Input: part model. Units: mm. Frame: model coordinates. Face numbers are marked on the shaded views. A direction names the side the tool comes from. Coordinates: 2 decimals unless noted, no trailing zeros. Loops run counter-clockwise (first coordinate to the right, second up) from the corner with the lowest first, then second, coordinate; pieces in that order, holes last. Notation, with made-up numbers: (26, -24) -> (77, -24) arc R36 ccw to (77, 13) -> close; hole circle Ø5 at (17, -23). An arc over 180 degrees is marked (long way). Put each result on its own line as item: value. Start each with the question number.
1) Contact query for flat-ended pins moving along their axis: P1, Ø7.5, axis at y = 9.5, z = 14.5, coming from the -X side; P2, Ø0.6, axis at x = 0, y = 8, coming from the -Z side; P3, Ø2, axis at x = 0, y = 4.5, coming from the -Z side; P4, Ø0.7, axis at x = -2, y = 6.5, coming from the +Z side. Output: stop coordinate, or through.
2) Material intervals for L1, parallel to Z at x = -2.05, y = 9.25; L2, parallel to Z at x = -0.75, y = 8.25; L3, parallel to X at y = 1.75, z = 7.5, sorted ascending.
3) Cut plane A-A (z = -7.5). Return the cut outline in (x, y), plus the area to 3 significant figures.
4) Pull-direction query (Z, two-part tool) for the marked faces 3, 4, 5 and 6; classes: pulls with the +Z half, pulls with the -Z half, needs draft (parallel to the pull), parting line crosses it, or undercut.
5) Set-up query: the marked faces 1 and 2. Return all of +Z, -Z, +X, -X, +Y, -Y with unobstructed straight access to the full face (end or side cutting, diameter ignored); none if empty.
Autodesk Inventor part; units mm, degrees
ref_plane "YZ Plane" through (0, 0, 0) normal (1, 0, 0) x (0, 1, 0)
ref_plane "XZ Plane" through (0, 0, 0) normal (0, 1, 0) x (-1, 0, 0)
ref_plane "XY Plane" through (0, 0, 0) normal (0, 0, 1) x (1, 0, 0)
sketch "Skizze1" plane through (0, 0, 0) normal (0, 1, 0) x (-1, 0, 0)
  line L0 (1.2301, 16.646) -> (-1.7699, 16.646)
  line L1 (-1.7699, 16.646) -> (-1.7699, 9.646)
  line L2 (-1.7699, 9.646) -> (1.2301, 9.646)
  line L3 (1.2301, 9.646) -> (1.2301, 16.646)
  line L4 (-1.7699, 9.646) -> (-0.5699, 9.646)
  line L5 (-0.5699, 9.646) -> (-0.5699, -20.354)
  line L6 (-0.5699, -20.354) -> (-1.7699, -20.354)
  line L7 (-1.7699, -20.354) -> (-1.7699, 9.646)
  line L8 (-0.5699, -20.354) -> (3.4301, -20.354)
  line L9 (3.4301, -20.354) -> (3.4301, -15.9771)
  line L10 (3.4301, -15.9771) -> (-0.5699, -15.9771)
  line L11 (-0.5699, -15.9771) -> (-0.5699, -20.354)
  point P0 (0, 0)
  dimension "d0" = 3
  dimension "d1" = 7
  dimension "d2" = 1.2
  dimension "d3" = 30
  dimension "d4" = 4
extrude "Extrusion1" add sketch "Skizze1" along normal blind 13
fillet "Rundung1" radius 4 1 edges at (1.7699, 6.5, -20.354)
sketch "Skizze2" plane through (0, 13, 0) normal (0, 1, 0) x (1, 0, 0)
  line L0 (0.5699, -9.646) -> (-1.2301, -9.646)
  line L1 (0.5699, -9.646) -> (-0.1301, -9.646)
  line L2 (-0.1301, -9.646) -> (-0.1301, -14.642)
  line L3 (-0.1301, -14.642) -> (0.5699, -14.642)
  line L4 (0.5699, -14.642) -> (0.5699, -9.646)
  point P0 (0, 0)
  point P1 (-0.3301, -9.646)
  point P2 (-0.1301, -9.646)
  dimension "d8" = 5
  dimension "d9" = 0.7
sketch "Skizze3" plane through (0, 13, 0) normal (0, 1, 0) x (1, 0, 0)
  line L0 (-3.4301, 20.354) -> (-3.4301, 15.9771)
  line L1 (-3.4301, 15.9771) -> (0.5699, 15.9771)
  arc A0 (0.5699, 15.9771) -> (-2.5715, 19.8839) centre (-3.4301, 15.9771) ccw
  line L2 (0.5699, 15.9771) -> (0.5699, -9.646)
  line L3 (0.5699, 15.9771) -> (-0.0301, 15.9771)
  arc A1 (-0.0301, 15.9771) -> (-2.8554, 19.3282) centre (-3.4301, 15.9771) ccw
  line L4 (-2.8554, 19.3282) -> (-2.5715, 19.8839)
  point P0 (0, 0)
  dimension "d10" = 0.6
extrude "Extrusion2" cut sketch "Skizze3" against normal blind 12
extrude "Extrusion3" cut sketch "Skizze2" against normal blind 12
sketch "Skizze4" plane through (-1.2301, 0, 9.646) normal (-1, 0, 0) x (0, 0, 1)
  line L0 (0, 0) -> (7, 0)
  line L1 (7, 0) -> (3.5, 0)
  line L2 (4.996, 13) -> (0, 13)
  line L3 (3.5, 13) -> (3.5, 0)
  line L4 (3.5, 6.5) -> (7, 6.5)
  line L5 (7, 0) -> (7, 13)
  circle A0 centre (3.5, 6.5) radius 1
  circle A1 centre (3.5, 1.1664) radius 1
  circle A2 centre (3.5, 3.7221) radius 1
  circle A3 centre (3.5, 8.9382) radius 1
  circle A4 centre (3.5, 11.2973) radius 1
  point P0 (-9.646, 0)
  dimension "d15" = 2
  dimension "d16" = 2
  dimension "d17" = 2
  dimension "d18" = 2
  dimension "d19" = 2
extrude "Extrusion4" add sketch "Skizze4" along normal blind 2.5 contours A4 L3 | L3 A4 | A3 L3 | L3 A3 | A1 L3 | L3 A1 | A0 L3 L4 | L4 L3 A0 | A2 L3 | L3 A2 | L3 A0
ref_plane "Arbeitsebene1" through (-1.2301, 11.2973, 14.146) normal (0, 0, 1) x (1, 0, 0)
sketch "Skizze5" plane through (-1.2301, 11.2973, 14.146) normal (0, 0, 1) x (1, 0, 0)
  line L0 (-2.2, -11.2973) -> (-2.2, 1.7027)
  ellipse E0 centre (-0.7, -4.7973) end of major axis (-0.7, -3.6152) minor radius 0.3015
  ellipse E1 centre (-0.7, -2.3523) end of major axis (-0.7, -1.125) minor radius 0.2616
  line L1 (0, -1.3591) -> (-2.5, -1.3591)
  ellipse E2 centre (-0.7, 0.0155) end of major axis (-0.7, 1.1416) minor radius 0.2973
  circle A0 centre (-1.25, -10.1312) radius 0.3762
  ellipse E3 centre (-0.7, -7.4834) end of major axis (-0.7, -8.7492) minor radius 0.3
  line L2 (0, -8.5752) -> (-2.5, -8.5752)
  point P0 (1.2301, -11.2973)
  point P1 (-0.8518, -8.5752)
  point P2 (-0.5482, -8.5752)
extrude "Extrusion5" cut sketch "Skizze5" against normal blind 1 contours E1 L1 | L1 E1 | E3 L2 | E0 | E2 picked at (-0.7898, -7.5169)
sketch "Skizze6" plane through (-1.2301, 11.2973, 14.146) normal (0, 0, 1) x (1, 0, 0)
  circle A0 centre (-1.315, -10.1413) radius 0.3946
  point P0 (1.2301, -11.2973)
extrude "Extrusion6" cut sketch "Skizze6" against normal blind 2.5
properties part number "hook_applicator_slide in"
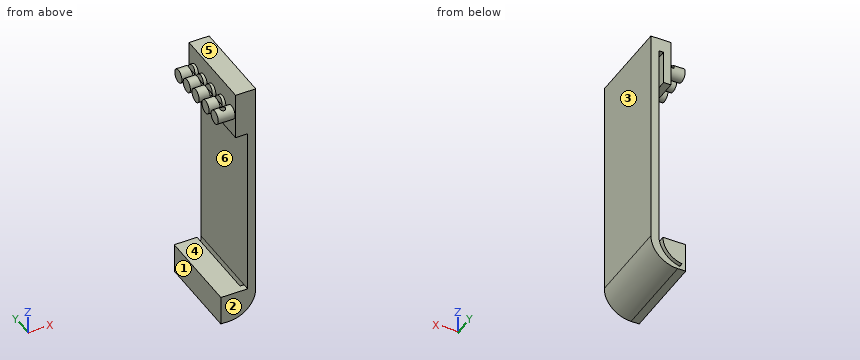
Results found:
1. P1: stops at x = -3.73
1. P2: stops at z = -19.86
1. P3: stops at z = -20.16
1. P4: stops at z = 14.15
2. L1: z = -20.35 to -19.73, -19.08 to -15.98, 12.2 to 13.15
2. L2: z = -20.07 to -18.95, -18.07 to -15.98, 9.65 to 16.65
2. L3: x = 0.57 to 1.77
3. outline: (0.57, 0) -> (1.77, 0) -> (1.77, 13) -> (0.57, 13) -> close
3. area: 15.6 mm2
4. face 3: needs draft
4. face 4: undercut
4. face 5: pulls with the +Z half
4. face 6: undercut
5. face 1: -Z, -X, +Y, -Y
5. face 2: +Z, -Z, +X, -X, -Y
